Source: CAD feature listing. Evaluate the final solid. Frame: model axes, mm. A direction names the side the tool comes from. Round coordinates to 2 decimals unless told otherwise and drop trailing zeros. Loops run counter-clockwise (first coordinate to the right, second up) from the corner with the lowest first, then second, coordinate; pieces in that order, holes last.
Item 1: Access query for faces 1 (the flat face through (6, 37, 0)), 2 (the flat face through (6, 30, 25.4)), 3 (the flat face through (0, 26, 13)), 4 (the flat face through (12.7, 26, 13)). Directions: +Z, -Z, +X, -X, +Y, -Y. A direction counts if a zero-diameter tool reaches every point of the face in a straight line with its end or side. Return the directions, or none.
Item 2: Section query C-C on y = 28. Return loops of the section in (x, z).
Item 3: First-contact query: P1, Ø1, axis at x = 4.5, z = 11.5, coming from the -Y side; P2, Ø3, axis at y = 31, z = 15.5, coming from the -X side; P3, Ø1, axis at x = -4.5, z = 5, coming from the -Y side. Flat tips, straight axial feed; report the tip coordinate or a pass-through.
Item 4: Ray query, L1, parallel to Z at x = 15, y = 57.5; L2, parallel to X at y = 13, z = 15.25; L3, parallel to Y at x = 7, z = 1.5. Return the intervals inside material, ascending.
Item 5: Section query B-B on z = 12.75. Return loops of the section in (x, y), then the cut area to 3 significant figures.
Item 6: Section query D-D on x = -7. Return loops of the section in (y, z).
Item 7: Section query A-A on x = 5. Return loops of the section in (y, z), then the cut area to 3 significant figures.
```python
from build123d import *

# Parameters (mm, degrees)
F1_DEPTH  = 25.4
F1_FACE_W = 40.370063592
F1_FACE_H = 25.4
F3_DEPTH  = 12.7
F5_DEPTH  = 25.4
F7_DEPTH  = 12.7
F9_DEPTH  = 12.7
F11_DEPTH = 12.7


with BuildPart() as f1:
    # F0 (on Top) → F1 (new body)
    with BuildSketch(Plane.XY):
        Polygon((0, 40.370063592), (0, 0), (12.7, 0), (12.7, 40.370063592), (25.4, 40.370063592), (25.4, 59.420063592), (-12.7, 59.420063592), (-12.7, 40.370063592), align=None)
    extrude(amount=F1_DEPTH)

    # F2 (on Right) + F1_face (on face) → F3 (cut)
    with BuildSketch(Plane.YZ):
        Polygon((8.6346566677, 25.5012921989), (0, 0), (13.8414995745, 0), (21.3624928147, 25.5012921989), align=None)
    with BuildSketch(Plane(origin=(0, 20.185031796, 12.7), x_dir=(0, -1, 0), z_dir=(-1, 0, 0))):
        Rectangle(F1_FACE_W, F1_FACE_H)
    extrude(amount=-F3_DEPTH, dir=(1, 0, 0), mode=Mode.SUBTRACT)

    # F4 (on face) → F5 (cut)
    with BuildSketch(Plane.YZ.offset(12.7)):
        Polygon((0, 0), (16.459165141, 25.4), (0, 25.4), align=None)
    extrude(amount=-F5_DEPTH, mode=Mode.SUBTRACT)

    # F6 (on face) → F7 (cut)
    with BuildSketch(Plane(origin=(-12.7, 0, 0), x_dir=(0, -1, 0), z_dir=(-1, 0, 0))):
        Polygon((-40.370063592, 25.4), (-49.895063592, 25.4), (-40.370063592, 0), align=None)
    extrude(amount=-F7_DEPTH, mode=Mode.SUBTRACT)

    # F8 (on Right) → F9 (join)
    with BuildSketch(Plane.YZ):
        Polygon((43.5419380665, 25.5644246936), (43.5981824994, 0), (52.4402596056, 25.5644246936), align=None)
    extrude(amount=F9_DEPTH)

    # F10 (on face) → F11 (cut)
    with BuildSketch(Plane.YZ.offset(25.4)):
        Polygon((40.370063592, 25.4), (40.370063592, 0), (49.895063592, 25.4), align=None)
    extrude(amount=-F11_DEPTH, mode=Mode.SUBTRACT)


solid = f1.part
```
Data:
1. face 1: -Z, +X, -X, +Y, -Y
1. face 2: +Z, +X, -X, -Y
1. face 3: +Z, -X, -Y
1. face 4: +Z, +X, -Y
2. outline: (0, 0) - (12.7, 0) - (12.7, 25.4) - (0, 25.4) - close
3. P1: stops at y = 7.13
3. P2: stops at x = 0
3. P3: stops at y = 42.06
4. L1: z = 0 to 25.4
4. L2: x = 0 to 12.7
4. L3: y = 0.97 to 59.42
5. outline: (-12.7, 45.15) - (0, 45.15) - (0, 8.26) - (12.7, 8.26) - (12.7, 45.15) - (25.4, 45.15) - (25.4, 59.42) - (-12.7, 59.42) - close
5. area: 1,010 mm2
6. outline: (40.37, 0) - (59.42, 0) - (59.42, 25.4) - (49.9, 25.4) - close
7. outline: (0, 0) - (59.42, 0) - (59.42, 25.4) - (52.38, 25.4) - (52.44, 25.56) - (43.54, 25.56) - (43.54, 25.4) - (16.46, 25.4) - close
7. area: 1,300 mm2
